Part model, mm, in its own coordinate system. A direction names the side the tool comes from. Give positions to 0.01 mm unless a question says otherwise; leave off trailing zeros. Write each loop counter-clockwise with the first axis right and the second up, starting at its lowest first coordinate (ties: lowest second). Pieces come first, ordered by that corner, then holes. Notation, with made-up numbers: (-14, 16.5) - (15, 16.5) arc R38 ccw to (15, 54.5) - close; hole circle Ø6 at (52.5, 26). An arc over 180 degrees is marked (long way). Answer in a Markdown table with one row per item. Add a question column.
1. Band-saw the part on C-C on z = 3. State how many separate pieces and enclosed holes the cut face has, plus the area to 3 significant figures.
2. Drop flat-ended pins along their axis: pin 1 Ø2 at (y, z) = (-26.45, 7.44) entering from -X; pin 2 Ø5 at (x, y) = (-132.5, -30) entering from +Z; pin 3 Ø5.5 at (x, y) = (-111.93, -24.59) entering from +Z. Give the stop position or say it passes through.
3. Band-saw the part on A-A on y = -12. Write the cut outline in (x, z) (3 decimals).
4. Band-saw the part on D-D on y = -42. Write the cut outline in (x, z) (3 decimals).
5. Pull direction X, two halves, no side cores. Call faces 5 (the cylindrical face through (-105.58, -24.45, 10.42)), 6 (the flat face through (-124, -24, 0)), 7 (the flat face through (-146.87, -5.2, 7.2)), 8 (the flat face through (-124, -24, 6.35)): released by +X, released by -X, zero draft, split by the parting line, or undercut.
6. Probe line 1 along Y through (x, z) = (-123, 4) (3 decimals); line 2 along X through (y, z) = (-14.5, 5.75); line 3 along Z through (x, y) = (-137, -19.5). List the from-to ranges inside material, lowest first.
7. Band-saw the part on B-B on x = -122.5. Write the cut outline in (y, z) (3 decimals).
8. Which spindle directions (+Z, -Z, +X, -X, +Y, -Y) get a long thin tool onto all of the face, cutting with end or side? Do faces 1 (the flat face through (-144.984, -26, 7)), 2 (the cylindrical face through (-109.472, -24.479, 3.131)), 3 (the flat face through (-136.354, -37.28, 10.42)), 4 (the flat face through (-113, -18.238, 7)). Say none if no direction does.
```python
from build123d import *

# Parameters (mm, degrees)
SKETCH1_W                 = 48.308864232
SKETCH1_H                 = 41.275
BOSS_EXTRUDE1_DEPTH       = 6.35
F_8_CLEARANCE_HOLE1_D     = 4.9149
F_1_4_CLEARANCE_HOLE1_D   = 7.14248
SKETCH9_W                 = 6.35
SKETCH9_H                 = 41.275
EXTRUDE_THIN1_DEPTH       = 8.255
CHAMFER2_SIZE             = 9.525
CUT_EXTRUDE1_DEPTH        = 156.127382276
CHAMFER1_SIZE             = 2.54
HOLE1_AT_2_COUNT          = 2
HOLE1_AT_2_PITCH          = 9.3599
F_2_CLEARANCE_HOLE1_D     = 2.7051
F_2_CLEARANCE_HOLE1_DEPTH = 3.175


with BuildPart() as part:
    # Sketch1 → Boss-Extrude1 (new body)
    with BuildSketch(Plane.XY):
        with Locations((-124.004465969, -24.5875)):
            Rectangle(SKETCH1_W, SKETCH1_H)
    extrude(amount=BOSS_EXTRUDE1_DEPTH)

    # #8 Clearance Hole1 (through all)
    with Locations(Plane.XY.offset(6.35)):
        with Locations((-111.927249911, -24.5875), (-136.081682027, -24.5875)):
            Hole(F_8_CLEARANCE_HOLE1_D / 2)

    # 1/4 Clearance Hole1 (through all)
    with Locations(Plane.XY.offset(6.35)):
        with Locations((-124.004465969, -14.4275), (-124.004465969, -34.7475)):
            Hole(F_1_4_CLEARANCE_HOLE1_D / 2)

    # Sketch9 → Extrude-Thin1 (add)
    with BuildSketch(Plane.XY.offset(6.35)):
        with Locations((-103.025033853, -24.5875)):
            Rectangle(SKETCH9_W, SKETCH9_H)
        with Locations((-144.983898085, -24.5875)):
            Rectangle(SKETCH9_W, SKETCH9_H)
    extrude(amount=EXTRUDE_THIN1_DEPTH)

    # Chamfer2
    # the kernel refuses this chamfer: 9.525 mm, written as the material it adds along each edge
    with BuildSketch(Plane(origin=(-106.200033853, -3.95, 6.35), x_dir=(0.0274958766105871, 0, 0.9996219169112966), z_dir=(0, -1, 0))) as chamfer2_piece_1_section:
        Polygon((CHAMFER2_SIZE * 0.999621916911, CHAMFER2_SIZE * 0.0274958766106), (-CHAMFER2_SIZE * 0.0274958766106, CHAMFER2_SIZE * 0.999621916911), (0, 0), align=None)
    chamfer2_piece_1 = extrude(amount=41.275, mode=Mode.PRIVATE)
    chamfer2_piece_1 = chamfer2_piece_1 - Plane(origin=(-111.927249911, -24.5875, 9.368765613), x_dir=(-1, 0, 0), z_dir=(0, 0, -1)) * Cylinder(2.45745, 121, mode=Mode.PRIVATE)
    chamfer2_piece_1 = split(chamfer2_piece_1, bisect_by=Plane(origin=(-109.341812124, -24.58749874, 14.605), z_dir=(0, 0, -1)), keep=Keep.TOP, mode=Mode.PRIVATE)
    add(chamfer2_piece_1)
    with BuildSketch(Plane(origin=(-141.808898085, -45.225, 6.35), x_dir=(0.9996219169112968, 0, -0.027495876610586386), z_dir=(0, 1, 0))) as chamfer2_piece_2_section:
        Polygon((CHAMFER2_SIZE * 0.999621916911, -CHAMFER2_SIZE * 0.0274958766106), (-CHAMFER2_SIZE * 0.0274958766106, -CHAMFER2_SIZE * 0.999621916911), (0, 0), align=None)
    chamfer2_piece_2 = extrude(amount=41.275, mode=Mode.PRIVATE)
    chamfer2_piece_2 = chamfer2_piece_2 - Plane(origin=(-136.081682027, -24.5875, 9.368765819), x_dir=(-1, 0, 0), z_dir=(0, 0, -1)) * Cylinder(2.45745, 121, mode=Mode.PRIVATE)
    chamfer2_piece_2 = split(chamfer2_piece_2, bisect_by=Plane(origin=(-138.667118685, -24.587501904, 14.605), z_dir=(0, 0, -1)), keep=Keep.TOP, mode=Mode.PRIVATE)
    add(chamfer2_piece_2)

    # Sketch10 → Cut-Extrude1 (cut, through all)
    with BuildSketch(Plane.XY.offset(6.35)):
        with BuildLine():
            Line((-136.081682027, -18.2375), (-111.927249911, -18.2375))
            ThreePointArc((-111.927249911, -18.2375), (-105.577249911, -24.5875), (-111.927249911, -30.9375))
            Line((-111.927249911, -30.9375), (-136.081682027, -30.9375))
            ThreePointArc((-136.081682027, -30.9375), (-142.431682027, -24.5875), (-136.081682027, -18.2375))
        make_face()
    extrude(amount=CUT_EXTRUDE1_DEPTH, mode=Mode.SUBTRACT)

    # Chamfer1
    chamfer1_edges = [part.edges().sort_by_distance(p)[0] for p in [
        (-99.850033853, -45.225, 7.3025),
        (-148.158898085, -45.225, 7.3025),
        (-148.158898085, -3.95, 7.3025),
        (-99.850033853, -3.95, 7.3025),
    ]]
    chamfer(chamfer1_edges, length=CHAMFER1_SIZE)

    # Sketch12 → Hole1 (revolve, cut)
    with BuildSketch(Plane(origin=(-148.158898085, -26.4544, 7.4422), x_dir=(0, 0, 1), z_dir=(0, 1, 0))):
        Polygon((0, 0), (0, 2.921), (1.4986, 2.921), (1.6383, 0), align=None)
    hole1 = revolve(axis=Axis((-38.158898085, -26.4544, 7.4422), (-1, 0, 0)), mode=Mode.SUBTRACT)

    # Hole1 at 2: Hole1 ×2
    with Locations(*[(0, i * HOLE1_AT_2_PITCH, 0) for i in range(1, HOLE1_AT_2_COUNT)]):
        add(hole1, mode=Mode.SUBTRACT)

    # #2 Clearance Hole1
    with Locations(Plane.ZY.offset(148.158898085)):
        with Locations((7.4422, -17.0945), (7.4422, -26.4544)):
            Hole(F_2_CLEARANCE_HOLE1_D / 2, depth=F_2_CLEARANCE_HOLE1_DEPTH)


solid = part.part
```
Values:
| question | item | result |
|---|---|---|
| 1 | separate pieces | 1 |
| 1 | enclosed holes | 4 |
| 1 | area | 1,860 mm² |
| 2 | pin 1 | stops at x = -144.98 |
| 2 | pin 2 | stops at z = 8.88 |
| 2 | pin 3 | stops at z = 6.35 |
| 3 | outline | (-148.159, 0) - (-126.624, 0) - (-126.624, 6.35) - (-132.284, 6.35) - (-140.539, 14.605) - (-148.159, 14.605) - close; (-121.385, 0) - (-99.85, 0) - (-99.85, 14.605) - (-107.47, 14.605) - (-115.725, 6.35) - (-121.385, 6.35) - close |
| 4 | outline | (-148.159, 0) - (-99.85, 0) - (-99.85, 14.605) - (-107.47, 14.605) - (-115.725, 6.35) - (-132.284, 6.35) - (-140.539, 14.605) - (-148.159, 14.605) - close |
| 5 | face 5 | undercut |
| 5 | face 6 | zero draft |
| 5 | face 7 | released by -X |
| 5 | face 8 | undercut |
| 6 | line 1 | y = -45.225 to -38.175, -31.32 to -17.855, -11 to -3.95 |
| 6 | line 2 | x = -148.16 to -127.57, -120.43 to -99.85 |
| 6 | line 3 | z = 0 to 6.35 |
| 7 | outline | (-45.225, 0) - (-37.986, 0) - (-37.986, 6.35) - (-45.225, 6.35) - close; (-31.509, 0) - (-17.666, 0) - (-17.666, 6.35) - (-31.509, 6.35) - close; (-11.189, 0) - (-3.95, 0) - (-3.95, 6.35) - (-11.189, 6.35) - close |
| 8 | face 1 | -X |
| 8 | face 2 | +Z, -Z |
| 8 | face 3 | +Z, +Y, -Y |
| 8 | face 4 | +Z |
